Build history of the part. All positions in model axes, mm. A direction names the side the tool comes from. Coordinates: 2 decimals unless noted, no trailing zeros. Order: outer loops, then holes, each group sorted by start corner. A loop starts at its lowest first (then second) coordinate and runs counter-clockwise, first axis right, second up. Notation, with made-up numbers: (47.25, 63.25) -> (105.25, 63.25) arc R24 cw to (105.25, 91.25) -> close; hole circle Ø9 at (58.25, 44). An arc over 180 degrees is marked (long way). Write each question's results on one line, items separated by ' | '.
from build123d import *

# Parameters (mm, degrees)
SCHIZZO1_R                   = 17.5
ESTRUSIONE_ESTRUSIONE1_DEPTH = 50
TAGLIO_ESTRUSIONE1_REACH     = 145.634
SCHIZZO10_R                  = 16.3
SKETCH2_R                    = 2.2
BOSS_EXTRUDE4_DEPTH          = 2


# Read off the part's stored shape, not the designer's step: Rivoluzione1
with BuildPart() as part:
    # Schizzo1 → Estrusione-Estrusione1 (new body)
    with BuildSketch(Plane(origin=(0, 0, 0), x_dir=(1, 0, 0), z_dir=(0, 1, 0))):
        with Locations(Location((0, 0, 0), (0, 0, 270))):
            Circle(SCHIZZO1_R)
    extrude(amount=ESTRUSIONE_ESTRUSIONE1_DEPTH)

    # Rivoluzione1 outline → Rivoluzione1 (revolve)
    with BuildSketch(Plane.XY):
        with BuildLine():
            Line((0, 141.485675179), (0, 136.5))
            Line((0, 136.5), (3.334103826, 136.5))
            add(Edge.make_bspline(
                [(3.334103826, 136.5), (16.3, 113.62789219), (16.3, 50)],
                knots=[0, 0, 0, 1, 1, 1], degree=2))
            Line((16.3, 50), (17.5, 50))
            add(Edge.make_bspline(
                [(17.5, 50), (17.5, 113.62789219), (2.55, 140)],
                knots=[0.063509007, 0.063509007, 0.063509007, 1.063509007, 1.063509007, 1.063509007], degree=2))
            ThreePointArc((2.55, 140), (1.475612649, 141.087167398), (0, 141.485675179))
        make_face()
    revolve(axis=Axis((0, 0, 0), (0, 1, 0)))

    # Schizzo10 → Taglio-Estrusione1 (cut, up to next)
    with BuildSketch(Plane(origin=(0, 0, 0), x_dir=(1, 0, 0), z_dir=(0, 1, 0)), mode=Mode.PRIVATE) as taglio_estrusione1_sk1:
        with Locations(Location((0, 0, 0), (0, 0, 270))):
            Circle(SCHIZZO10_R)
    taglio_estrusione1_tool1 = extrude(taglio_estrusione1_sk1.sketch, amount=TAGLIO_ESTRUSIONE1_REACH, mode=Mode.PRIVATE) & part.part
    add(taglio_estrusione1_tool1.solids().sort_by_distance((0, 0, 0))[0], mode=Mode.SUBTRACT)

    # Sketch2 → Boss-Extrude4 (add)
    # profile 1 of 2: a face of its own
    with BuildSketch(Plane.XZ):
        with BuildLine():
            ThreePointArc((8.3, 4.5), (3.8, 0), (8.3, -4.5))
            Line((8.3, -4.5), (15.666524822, -4.5))
            ThreePointArc((15.666524822, -4.5), (16.3, 0), (15.666524822, 4.5))
            Line((15.666524822, 4.5), (8.3, 4.5))
        make_face()
        with Locations(Location((8.3, 0, 0), (0, 0, 270))):
            Circle(SKETCH2_R, mode=Mode.SUBTRACT)
    # profile 2 of 2: a face of its own
    with BuildSketch(Plane.XZ):
        with BuildLine():
            Line((-8.3, 4.5), (-15.666524822, 4.5))
            ThreePointArc((-15.666524822, 4.5), (-16.3, 0), (-15.666524822, -4.5))
            Line((-15.666524822, -4.5), (-8.3, -4.5))
            ThreePointArc((-8.3, -4.5), (-3.8, 0), (-8.3, 4.5))
        make_face()
        with Locations(Location((-8.3, 0, 0), (0, 0, 270))):
            Circle(SKETCH2_R, mode=Mode.SUBTRACT)
    extrude(amount=-BOSS_EXTRUDE4_DEPTH)


solid = part.part
Item 1: Tool access for faces 1 (the cylindrical face through (4.896, 24.65, 15.547)), 2 (the cylindrical face through (-10.448, 0.986, 0.477)): list every direction of +Z, -Z, +X, -X, +Y, -Y with a clear straight run to the whole face (end or side of a thin tool).
Answer:
face 1: none | face 2: -Y
Item 2: Pull direction Z, two halves, no side cores. Call faces 3 (the cylindrical face through (-10.648, 24.65, -13.887)), 4 (the flat face through (4, 0, 0)), 5 (the flat face through (-12, 2, 0)): released by +Z, released by -Z, zero draft, split by the parting line, or undercut.
Answer:
face 3: split by the parting line | face 4: zero draft | face 5: undercut
Item 3: Slice it at B-B, the plane z = 0. State how many separate pieces and enclosed holes the cut face has, and give its area (3 significant figures).
Answer:
separate pieces: 3 | enclosed holes: 0 | area: 348 mm^2
Item 4: Drill centre lines: line 1 (X direction, y = 0.45, z = 0); line 2 (Z direction, x = 0, y = 23.5); line 3 (Z direction, x = -2.5, y = 72). Where is each one in solid material? Low to high. Write a range as from..to.
Answer:
line 1: x = -17.5..-10.5, -6.1..-3.8, 3.8..6.1, 10.5..17.5 | line 2: z = -17.5..-16.3, 16.3..17.5 | line 3: z = -16.82..-15.66, 15.66..16.82
Item 5: Pin check, flat tips, straight feed: pin 1 (2 mm diameter, centred on x = 10.5, y = 0.5, fed in from -Z); pin 2 (12 mm diameter, centred on x = 2, z = 9, fed in from +Y); pin 3 (5.5 mm diameter, centred on x = -1, z = 1, fed in from -Y). Stop position of each tip, or through.
Answer:
pin 1: stops at z = -14.7 | pin 2: stops at y = 138.79 | pin 3: stops at y = 134.97
Item 6: Slice it at A-A, the plane y = 41. List the corners of the cut face in (x, z), and give its area (3 significant figures).
Answer:
outline: circle Ø35 at (0, 0); hole circle Ø32.6 at (0, 0) | area: 127 mm^2
